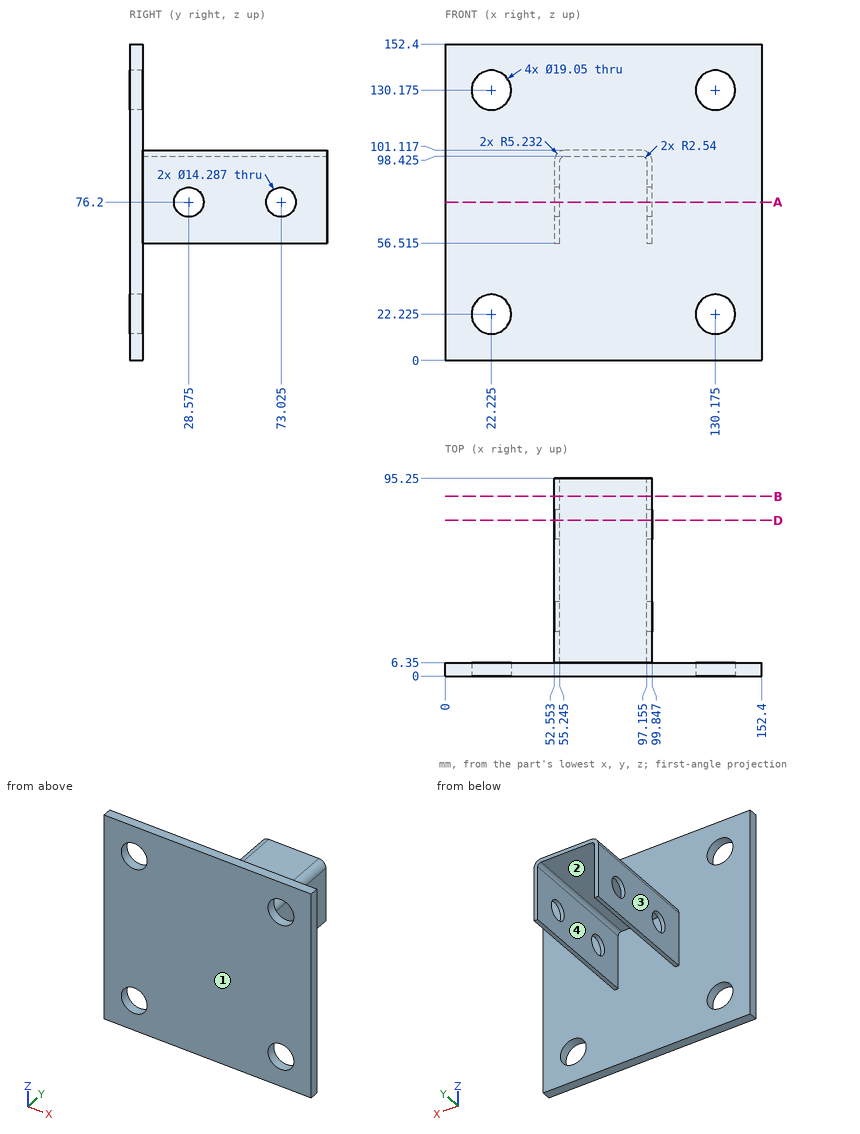
Part print with two shaded views. Sizes in mm from the minimum x, y, z corner. Coordinates: 2 decimals unless noted, no trailing zeros. Write each loop counter-clockwise with the first axis right and the second up, starting at its lowest first coordinate (ties: lowest second). Pieces come first, ordered by that corner, then holes.
(1) Cut at B-B on y = 86.5. List the corners of the cut face in (x, z) (1 decimal).
(2) Pin check, flat tips, straight feed: pin 1 Ø17 at (x, z) = (130.175, 22.225) entering from -Y; pin 2 Ø3 at (x, z) = (50.5, 87.5) entering from +Y; pin 3 Ø0.8 at (x, y) = (53.5, 39) entering from -Z (1 decimal); pin 4 Ø23 at (y, z) = (28.575, 76.2) entering from +X. Stop position of each tip, or through.
(3) Drill centre lines: line 1 (Y direction, x = 99.3, z = 76.2); line 2 (X direction, y = 89.5, z = 73.5) (1 decimal); line 3 (Y direction, x = 57, z = 109.5). Where is each one in solid material? Low to high.
(4) Cut at D-D on y = 75. List the corners of the cut face in (x, z) (1 decimal).
(5) Mould opens along X. For the marked faces 1, 2, 3 and 4 say: pulls with the +X half, pulls with the -X half, needs draft (parallel to the pull), parting line crosses it, or undercut.
(6) Cut at A-A on z = 76.2. State how many separate pieces and enclosed holes the cut face has, and give its area (3 significant figures).
Working result:
1. outline: (52.6, 56.5) - (55.2, 56.5) - (55.2, 95.9) arc R2.5 cw to (57.8, 98.4) - (94.6, 98.4) arc R2.5 cw to (97.2, 95.9) - (97.2, 56.5) - (99.8, 56.5) - (99.8, 95.9) arc R5.2 ccw to (94.6, 101.1) - (57.8, 101.1) arc R5.2 ccw to (52.6, 95.9) - close
2. pin 1: passes through
2. pin 2: stops at y = 6.35
2. pin 3: stops at z = 56.5
2. pin 4: stops at x = 99.85
3. line 1: y = 0 to 21.43, 35.72 to 65.88, 80.17 to 95.25
3. line 2: x = 52.6 to 55.2, 97.2 to 99.8
3. line 3: y = 0 to 6.35
4. outline: (52.6, 56.5) - (55.2, 56.5) - (55.2, 69.3) - (52.6, 69.3) - close; (52.6, 83.1) - (55.2, 83.1) - (55.2, 95.9) arc R2.5 cw to (57.8, 98.4) - (94.6, 98.4) arc R2.5 cw to (97.2, 95.9) - (97.2, 83.1) - (99.8, 83.1) - (99.8, 95.9) arc R5.2 ccw to (94.6, 101.1) - (57.8, 101.1) arc R5.2 ccw to (52.6, 95.9) - close; (97.2, 56.5) - (99.8, 56.5) - (99.8, 69.3) - (97.2, 69.3) - close
5. face 1: needs draft
5. face 2: undercut
5. face 3: pulls with the -X half
5. face 4: undercut
6. separate pieces: 5
6. enclosed holes: 0
6. area: 1,290 mm2
